from build123d import *

# Parameters (mm, degrees)
ESQUISSE1_R        = 8
ESQUISSE1_W        = 6
ESQUISSE1_H        = 4.95
BOSS_EXTRU_1_DEPTH = 6


with BuildPart() as part:
    # Esquisse1 → Boss.-Extru.1 (new body)
    with BuildSketch(Plane.XY):
        Polygon((-12, 0), (12, 0), (12, -0.2), (12, -5), (18, -5), (18, -10.2), (12, -10.2), (12, -15), (18, -15), (18, -20.2), (12, -20.2), (12, -25), (18, -25), (18, -30.2), (12, -30.2), (12, -35), (18, -35), (18, -115), (15.9, -115), (15.9, -110.05), (9.9, -110.05), (9.9, -115), (-9.9, -115), (-9.9, -110.05), (-15.9, -110.05), (-15.9, -115), (-18, -115), (-18, -35), (-12, -35), (-12, -30.2), (-18, -30.2), (-18, -25), (-12, -25), (-12, -20.2), (-18, -20.2), (-18, -15), (-12, -15), (-12, -10.2), (-18, -10.2), (-18, -5), (-12, -5), (-12, -0.2), align=None)
        with Locations((1, -87.7)):
            Circle(ESQUISSE1_R, mode=Mode.SUBTRACT)
        with Locations((1, -62)):
            Circle(ESQUISSE1_R, mode=Mode.SUBTRACT)
        with Locations((-12.9, -102.525)):
            Rectangle(ESQUISSE1_W, ESQUISSE1_H, mode=Mode.SUBTRACT)
        with Locations((12.9, -102.525)):
            Rectangle(ESQUISSE1_W, ESQUISSE1_H, mode=Mode.SUBTRACT)
    extrude(amount=BOSS_EXTRU_1_DEPTH)


solid = part.part
Check sheet for the modelled part. Datum: model origin and axes. Units: mm. A direction names the side the tool comes from. Give positions to 0.01 mm unless a question says otherwise; leave off trailing zeros. Write each loop counter-clockwise with the first axis right and the second up, starting at its lowest first coordinate (ties: lowest second). Pieces come first, ordered by that corner, then holes. Notation, with made-up numbers: (80.25, -27.75) -> (113.25, -27.75) arc R20 cw to (113.25, -3.75) -> close; hole circle Ø2 at (-27.5, 16.5). An arc over 180 degrees is marked (long way). One line per item, written item: value. Start each with the question number.
Item 1: Draft check along Y on faces 1 (the flat face through (9.9, -103, 3)), 2 (the flat face through (-18, -18, 3)), 3 (the flat face through (-13, -110.05, 3)). Enter one of: +Y half, -Y half, draft (parallel to the pull), parting line (faces both ways), or undercut.
Item 2: Section check A-A on y = -87.7. Record the cut outline in (x, z).
Item 3: Material ranges on probe 1 along Y at (x, z) = (1.5, 1.45); probe 2 along Y at (x, z) = (-14, 1.6); probe 3 along Y at (x, z) = (6.5, 5.55), recorded low to high. Write a range as from..to.
Item 4: Section check B-B on x = 1. Record the cut outline in (y, z), then the cut area to 3 significant figures.
Item 5: Gauge pin test, flat ends, axial feed: pin 1 (3 mm diameter, centred on x = 15.5, z = 4.5, fed in from -Y); pin 2 (3 mm diameter, centred on x = -13.5, z = 4.5, fed in from -Y); pin 3 (2.5 mm diameter, centred on y = -22.5, z = 3.5, fed in from +X); pin 4 (1.4 mm diameter, centred on y = -32.5, z = 4, fed in from -X). Record the tip position at first contact, or that the pin passes through.
Item 6: Section check C-C on z = 3.4. State how many separate pieces and enclosed holes the cut face has, then the cut area to 3 significant figures.
Item 7: Tool access check on faces 4 (the flat face through (-12, -2, 3)), 5 (the flat face through (12, -13, 3)), 6 (the flat face through (18, -8, 3)), 7 (the flat face through (15.9, -113, 3)), 8 (the flat face through (-12, -23, 3)). Record the directions out of +Z, -Z, +X, -X, +Y, -Y that give a thin tool (end or side, any length) a straight path to the whole face; none if there is none.
Item 8: Section check D-D on y = -14. Record the cut outline in (x, z), then the cut area to 3 significant figures.
Results list:
1. face 1: undercut
1. face 2: draft
1. face 3: -Y half
2. outline: (-18, 0) -> (-7, 0) -> (-7, 6) -> (-18, 6) -> close; (9, 0) -> (18, 0) -> (18, 6) -> (9, 6) -> close
3. probe 1: -115..-95.68, -79.72..-69.98, -54.02..0
3. probe 2: -110.05..-105, -100.05..-35, -30.2..-25, -20.2..-15, -10.2..-5
3. probe 3: -115..-93.51, -81.89..-67.81, -56.19..0
4. outline: (-115, 0) -> (-95.7, 0) -> (-95.7, 6) -> (-115, 6) -> close; (-79.7, 0) -> (-70, 0) -> (-70, 6) -> (-79.7, 6) -> close; (-54, 0) -> (0, 0) -> (0, 6) -> (-54, 6) -> close
4. area: 498 mm²
5. pin 1: y = -115
5. pin 2: y = -110.05
5. pin 3: x = 12
5. pin 4: x = -12
6. separate pieces: 1
6. enclosed holes: 4
6. area: 3,390 mm²
7. face 4: +Z, -Z, -X, +Y
7. face 5: +Z, -Z, +X
7. face 6: +Z, -Z, +X, +Y, -Y
7. face 7: +Z, -Z, -Y
7. face 8: +Z, -Z, -X
8. outline: (-12, 0) -> (12, 0) -> (12, 6) -> (-12, 6) -> close
8. area: 144 mm²
